from build123d import *

# Parameters (mm, degrees)
BOSS_EXTRUDE1_DEPTH = 20
CUT_EXTRUDE1_REACH  = 28.881
CIRPATTERN1_COUNT   = 2
CIRPATTERN1_ANGLE   = 90


with BuildPart() as part:
    # Sketch1 → Boss-Extrude1 (new body)
    with BuildSketch(Plane.XY):
        Polygon((0, 0), (0, 12.7), (1.58, 12.7), (1.58, 1.58), (12.7, 1.58), (12.7, 0), align=None)
    extrude(amount=BOSS_EXTRUDE1_DEPTH)

    # Sketch2 → Cut-Extrude1 (cut, up to next)
    with BuildSketch(Plane.ZY, mode=Mode.PRIVATE) as cut_extrude1_sk1:
        with BuildLine():
            ThreePointArc((4, 7.14), (5, 6.14), (6, 7.14))
            Line((6, 7.14), (4, 7.14))
        make_face()
    cut_extrude1_tool1 = extrude(cut_extrude1_sk1.sketch, amount=-CUT_EXTRUDE1_REACH, mode=Mode.PRIVATE) & part.part
    # Sketch2 → Cut-Extrude1 (cut, up to next)
    with BuildSketch(Plane.ZY, mode=Mode.PRIVATE) as cut_extrude1_sk2:
        with BuildLine():
            Line((4, 7.14), (6, 7.14))
            ThreePointArc((6, 7.14), (5, 8.14), (4, 7.14))
        make_face()
    cut_extrude1_tool2 = extrude(cut_extrude1_sk2.sketch, amount=-CUT_EXTRUDE1_REACH, mode=Mode.PRIVATE) & part.part
    # Sketch2 → Cut-Extrude1 (cut, up to next)
    with BuildSketch(Plane.ZY, mode=Mode.PRIVATE) as cut_extrude1_sk3:
        with BuildLine():
            ThreePointArc((4, 7.14), (5, 6.14), (6, 7.14))
            Line((6, 7.14), (4, 7.14))
        make_face()
    cut_extrude1_tool3 = extrude(cut_extrude1_sk3.sketch, amount=-CUT_EXTRUDE1_REACH, mode=Mode.PRIVATE) & part.part
    # Sketch2 → Cut-Extrude1 (cut, up to next)
    with BuildSketch(Plane.ZY, mode=Mode.PRIVATE) as cut_extrude1_sk4:
        with BuildLine():
            Line((4, 7.14), (6, 7.14))
            ThreePointArc((6, 7.14), (5, 8.14), (4, 7.14))
        make_face()
    cut_extrude1_tool4 = extrude(cut_extrude1_sk4.sketch, amount=-CUT_EXTRUDE1_REACH, mode=Mode.PRIVATE) & part.part
    # Sketch2 → Cut-Extrude1 (cut, up to next)
    with BuildSketch(Plane.ZY, mode=Mode.PRIVATE) as cut_extrude1_sk5:
        with BuildLine():
            ThreePointArc((16, 7.14), (15, 8.14), (14, 7.14))
            Line((14, 7.14), (16, 7.14))
        make_face()
    cut_extrude1_tool5 = extrude(cut_extrude1_sk5.sketch, amount=-CUT_EXTRUDE1_REACH, mode=Mode.PRIVATE) & part.part
    # Sketch2 → Cut-Extrude1 (cut, up to next)
    with BuildSketch(Plane.ZY, mode=Mode.PRIVATE) as cut_extrude1_sk6:
        with BuildLine():
            Line((16, 7.14), (14, 7.14))
            ThreePointArc((14, 7.14), (15, 6.14), (16, 7.14))
        make_face()
    cut_extrude1_tool6 = extrude(cut_extrude1_sk6.sketch, amount=-CUT_EXTRUDE1_REACH, mode=Mode.PRIVATE) & part.part
    # Sketch2 → Cut-Extrude1 (cut, up to next)
    with BuildSketch(Plane.ZY, mode=Mode.PRIVATE) as cut_extrude1_sk7:
        with BuildLine():
            ThreePointArc((16, 7.14), (15, 8.14), (14, 7.14))
            Line((14, 7.14), (16, 7.14))
        make_face()
    cut_extrude1_tool7 = extrude(cut_extrude1_sk7.sketch, amount=-CUT_EXTRUDE1_REACH, mode=Mode.PRIVATE) & part.part
    # Sketch2 → Cut-Extrude1 (cut, up to next)
    with BuildSketch(Plane.ZY, mode=Mode.PRIVATE) as cut_extrude1_sk8:
        with BuildLine():
            Line((16, 7.14), (14, 7.14))
            ThreePointArc((14, 7.14), (15, 6.14), (16, 7.14))
        make_face()
    cut_extrude1_tool8 = extrude(cut_extrude1_sk8.sketch, amount=-CUT_EXTRUDE1_REACH, mode=Mode.PRIVATE) & part.part
    cut_extrude1_1 = cut_extrude1_tool1.solids().sort_by_distance((0, 6.715587, 5))[0]
    add(cut_extrude1_1, mode=Mode.SUBTRACT)
    cut_extrude1_2 = cut_extrude1_tool2.solids().sort_by_distance((0, 7.564413, 5))[0]
    add(cut_extrude1_2, mode=Mode.SUBTRACT)
    cut_extrude1_3 = cut_extrude1_tool3.solids().sort_by_distance((0, 6.715587, 5))[0]
    add(cut_extrude1_3, mode=Mode.SUBTRACT)
    cut_extrude1_4 = cut_extrude1_tool4.solids().sort_by_distance((0, 7.564413, 5))[0]
    add(cut_extrude1_4, mode=Mode.SUBTRACT)
    cut_extrude1_5 = cut_extrude1_tool5.solids().sort_by_distance((0, 7.564413, 15))[0]
    add(cut_extrude1_5, mode=Mode.SUBTRACT)
    cut_extrude1_6 = cut_extrude1_tool6.solids().sort_by_distance((0, 6.715587, 15))[0]
    add(cut_extrude1_6, mode=Mode.SUBTRACT)
    cut_extrude1_7 = cut_extrude1_tool7.solids().sort_by_distance((0, 7.564413, 15))[0]
    add(cut_extrude1_7, mode=Mode.SUBTRACT)
    cut_extrude1_8 = cut_extrude1_tool8.solids().sort_by_distance((0, 6.715587, 15))[0]
    add(cut_extrude1_8, mode=Mode.SUBTRACT)
    cut_extrude1 = cut_extrude1_1 + cut_extrude1_2 + cut_extrude1_3 + cut_extrude1_4 + cut_extrude1_5 + cut_extrude1_6 + cut_extrude1_7 + cut_extrude1_8  # Cut-Extrude1 as one shape, for the pattern or mirror that repeats it

    # CirPattern1: Cut-Extrude1; each copy of Cut-Extrude1 runs up to whatever stops it at its own place
    cirpattern1_before = part.part  # the part as the pattern finds it: every copy runs up to it
    cirpattern1_cut_extrude1_long1 = extrude(cut_extrude1_sk1.sketch, amount=-CUT_EXTRUDE1_REACH, mode=Mode.PRIVATE)
    cirpattern1_cut_extrude1_long2 = extrude(cut_extrude1_sk2.sketch, amount=-CUT_EXTRUDE1_REACH, mode=Mode.PRIVATE)
    cirpattern1_cut_extrude1_long3 = extrude(cut_extrude1_sk3.sketch, amount=-CUT_EXTRUDE1_REACH, mode=Mode.PRIVATE)
    cirpattern1_cut_extrude1_long4 = extrude(cut_extrude1_sk4.sketch, amount=-CUT_EXTRUDE1_REACH, mode=Mode.PRIVATE)
    cirpattern1_cut_extrude1_long5 = extrude(cut_extrude1_sk5.sketch, amount=-CUT_EXTRUDE1_REACH, mode=Mode.PRIVATE)
    cirpattern1_cut_extrude1_long6 = extrude(cut_extrude1_sk6.sketch, amount=-CUT_EXTRUDE1_REACH, mode=Mode.PRIVATE)
    cirpattern1_cut_extrude1_long7 = extrude(cut_extrude1_sk7.sketch, amount=-CUT_EXTRUDE1_REACH, mode=Mode.PRIVATE)
    cirpattern1_cut_extrude1_long8 = extrude(cut_extrude1_sk8.sketch, amount=-CUT_EXTRUDE1_REACH, mode=Mode.PRIVATE)
    cirpattern1_cut_extrude1_tool1_1 = cirpattern1_cut_extrude1_long1.rotate(Axis((1.58, 1.58, 20), (0, 0, -1)), 1 * CIRPATTERN1_ANGLE / (CIRPATTERN1_COUNT - 1)) & cirpattern1_before
    add(cirpattern1_cut_extrude1_tool1_1.solids().sort_by_distance((6.715587, 3.16, 5))[0], mode=Mode.SUBTRACT)
    cirpattern1_cut_extrude1_tool2_1 = cirpattern1_cut_extrude1_long2.rotate(Axis((1.58, 1.58, 20), (0, 0, -1)), 1 * CIRPATTERN1_ANGLE / (CIRPATTERN1_COUNT - 1)) & cirpattern1_before
    add(cirpattern1_cut_extrude1_tool2_1.solids().sort_by_distance((7.564413, 3.16, 5))[0], mode=Mode.SUBTRACT)
    cirpattern1_cut_extrude1_tool3_1 = cirpattern1_cut_extrude1_long3.rotate(Axis((1.58, 1.58, 20), (0, 0, -1)), 1 * CIRPATTERN1_ANGLE / (CIRPATTERN1_COUNT - 1)) & cirpattern1_before
    add(cirpattern1_cut_extrude1_tool3_1.solids().sort_by_distance((6.715587, 3.16, 5))[0], mode=Mode.SUBTRACT)
    cirpattern1_cut_extrude1_tool4_1 = cirpattern1_cut_extrude1_long4.rotate(Axis((1.58, 1.58, 20), (0, 0, -1)), 1 * CIRPATTERN1_ANGLE / (CIRPATTERN1_COUNT - 1)) & cirpattern1_before
    add(cirpattern1_cut_extrude1_tool4_1.solids().sort_by_distance((7.564413, 3.16, 5))[0], mode=Mode.SUBTRACT)
    cirpattern1_cut_extrude1_tool5_1 = cirpattern1_cut_extrude1_long5.rotate(Axis((1.58, 1.58, 20), (0, 0, -1)), 1 * CIRPATTERN1_ANGLE / (CIRPATTERN1_COUNT - 1)) & cirpattern1_before
    add(cirpattern1_cut_extrude1_tool5_1.solids().sort_by_distance((7.564413, 3.16, 15))[0], mode=Mode.SUBTRACT)
    cirpattern1_cut_extrude1_tool6_1 = cirpattern1_cut_extrude1_long6.rotate(Axis((1.58, 1.58, 20), (0, 0, -1)), 1 * CIRPATTERN1_ANGLE / (CIRPATTERN1_COUNT - 1)) & cirpattern1_before
    add(cirpattern1_cut_extrude1_tool6_1.solids().sort_by_distance((6.715587, 3.16, 15))[0], mode=Mode.SUBTRACT)
    cirpattern1_cut_extrude1_tool7_1 = cirpattern1_cut_extrude1_long7.rotate(Axis((1.58, 1.58, 20), (0, 0, -1)), 1 * CIRPATTERN1_ANGLE / (CIRPATTERN1_COUNT - 1)) & cirpattern1_before
    add(cirpattern1_cut_extrude1_tool7_1.solids().sort_by_distance((7.564413, 3.16, 15))[0], mode=Mode.SUBTRACT)
    cirpattern1_cut_extrude1_tool8_1 = cirpattern1_cut_extrude1_long8.rotate(Axis((1.58, 1.58, 20), (0, 0, -1)), 1 * CIRPATTERN1_ANGLE / (CIRPATTERN1_COUNT - 1)) & cirpattern1_before
    add(cirpattern1_cut_extrude1_tool8_1.solids().sort_by_distance((6.715587, 3.16, 15))[0], mode=Mode.SUBTRACT)


solid = part.part
Read the model definition and answer for the solid it produces. Units are mm, in the model's axes. A direction names the side the tool comes from. Coordinates: 2 decimals unless noted, no trailing zeros. Order: outer loops, then holes, each group sorted by start corner. A loop starts at its lowest first (then second) coordinate and runs counter-clockwise, first axis right, second up. Notation, with made-up numbers: (20, 47.25) - (40, 47.25) arc R34 cw to (40, 78.25) - close; hole circle Ø8 at (-29, -40). An arc over 180 degrees is marked (long way). Use one line per item in the form item = value.
(1) Section D-D, the plane z = 8 is taken. Give the vertices of the cut face in (x, y).
Computed values:
outline = (0, 0) - (12.7, 0) - (12.7, 1.58) - (1.58, 1.58) - (1.58, 12.7) - (0, 12.7) - close
(2) For a pull along X with two mould halves and no side action, classify faces 1 (the face through (1.58, 7, 10)), 2 (the face through (6.84, 0.801, 14.046)), 3 (the face through (6, 0, 10)), 4 (the face through (6.15, 0.8, 5.13)) as pulls with the +X half, pulls with the -X half, needs draft (parallel to the pull), parting line crosses it, or undercut.
Computed values:
face_1 = pulls with the +X half
face_2 = undercut
face_3 = needs draft
face_4 = undercut
(3) Section A-A, the plane y = 7.14 is taken. Give the vertices of the cut face in (x, z).
Computed values:
outline = (0, 0) - (1.58, 0) - (1.58, 4) - (0, 4) - close; (0, 6) - (1.58, 6) - (1.58, 14) - (0, 14) - close; (0, 16) - (1.58, 16) - (1.58, 20) - (0, 20) - close
(4) Section C-C, the plane z = 15 is taken. Give the vertices of the cut face in (x, y).
Computed values:
outline = (0, 0) - (6.14, 0) - (6.14, 1.58) - (1.58, 1.58) - (1.58, 6.14) - (0, 6.14) - close; (0, 8.14) - (1.58, 8.14) - (1.58, 12.7) - (0, 12.7) - close; (8.14, 0) - (12.7, 0) - (12.7, 1.58) - (8.14, 1.58) - close
(5) Given pin 1 Ø2.5 at (y, z) = (7.14, 15) entering from +X, flat-ended and moving along its own axis, determine where the tip first touches the part or whether it passes through.
Computed values:
pin_1 = 1.58
(6) Which of the six approach directions +Z, -Z, +X, -X, +Y, -Y give full straight-line access (tool end or side, diameter ignored) to faces 5 (the face through (7, 1.58, 10)), 6 (the face through (4, 1, 20))?
Computed values:
face_5 = +Z, -Z, +X, +Y
face_6 = +Z, +X, -X, +Y, -Y
(7) Straight lines are drawn through the part: L1, parallel to X at y = 0.75, z = 5; L2, parallel to X at y = 3.25, z = 4. For each, find the intervals that lie inside material, in ascending order.
Computed values:
L1 = 0 to 6.14, 8.14 to 12.7
L2 = 0 to 1.58
